Input: part model. Units: mm. Frame: model coordinates. Face numbers are marked on the shaded views. A direction names the side the tool comes from. Coordinates: 2 decimals unless noted, no trailing zeros. Loops run counter-clockwise (first coordinate to the right, second up) from the corner with the lowest first, then second, coordinate; pieces in that order, holes last.
```python
from build123d import *

# Parameters (mm, degrees)
SKETCH1_R            = 3.5
SKETCH1_R_2          = 8
BOSS_EXTRUDE1_DEPTH  = 10
CUT_EXTRUDE1_DEPTH   = 5
FILLET1_R            = 2
SKETCH3_R            = 12.5
CUT_EXTRUDE2_DEPTH   = 10
FILLET1_OF_MIRROR1_R = 2
SKETCH6_R            = 3
CUT_EXTRUDE3_DEPTH   = 10


with BuildPart() as part:
    # Sketch1 → Boss-Extrude1 (new, symmetric)
    # profile 1 of 2: a face of its own
    with BuildSketch(Plane(origin=(0, 0, 0), x_dir=(0, 0, -1), z_dir=(1, 0, 0))):
        with BuildLine():
            ThreePointArc((-46, 62.5), (0, 108.5), (46, 62.5))
            Line((46, 62.5), (46, -62.5))
            Line((46, -62.5), (-46, -62.5))
            Line((-46, -62.5), (-46, 62.5))
        make_face()
        with Locations((-33.774990748, 82)):
            Circle(SKETCH1_R, mode=Mode.SUBTRACT)
        with Locations((-33.774990748, 43)):
            Circle(SKETCH1_R, mode=Mode.SUBTRACT)
        with Locations((0, 23.5)):
            Circle(SKETCH1_R, mode=Mode.SUBTRACT)
        with Locations((33.774990748, 43)):
            Circle(SKETCH1_R, mode=Mode.SUBTRACT)
        with Locations((33.774990748, 82)):
            Circle(SKETCH1_R, mode=Mode.SUBTRACT)
        with Locations((0, 62.5)):
            Circle(SKETCH1_R_2, mode=Mode.SUBTRACT)
        with Locations((0, 101.5)):
            Circle(SKETCH1_R, mode=Mode.SUBTRACT)
        with BuildLine():
            ThreePointArc((-25.103448276, 16.960820334), (-31.051285766, 16.872502771), (-34, 11.706299603))
            Line((-34, 11.706299603), (-34, -44.5))
            ThreePointArc((-34, -44.5), (-32.242640687, -48.742640687), (-28, -50.5))
            Line((-28, -50.5), (28, -50.5))
            ThreePointArc((28, -50.5), (32.242640687, -48.742640687), (34, -44.5))
            Line((34, -44.5), (34, 11.706299603))
            ThreePointArc((34, 11.706299603), (31.051285766, 16.872502771), (25.103448276, 16.960820334))
            ThreePointArc((25.103448276, 16.960820334), (0, 10.5), (-25.103448276, 16.960820334))
        make_face(mode=Mode.SUBTRACT)
    # profile 2 of 2: a face of its own
    with BuildSketch(Plane(origin=(0, 0, 0), x_dir=(0, 0, -1), z_dir=(1, 0, 0))):
        with BuildLine():
            ThreePointArc((-25.103448276, 16.960820334), (0, 10.5), (25.103448276, 16.960820334))
            ThreePointArc((25.103448276, 16.960820334), (31.051285766, 16.872502771), (34, 11.706299603))
            Line((34, 11.706299603), (34, -44.5))
            ThreePointArc((34, -44.5), (32.242640687, -48.742640687), (28, -50.5))
            Line((28, -50.5), (-28, -50.5))
            ThreePointArc((-28, -50.5), (-32.242640687, -48.742640687), (-34, -44.5))
            Line((-34, -44.5), (-34, 11.706299603))
            ThreePointArc((-34, 11.706299603), (-31.051285766, 16.872502771), (-25.103448276, 16.960820334))
        make_face()
    extrude(amount=BOSS_EXTRUDE1_DEPTH, both=True)

    # Sketch2 → Cut-Extrude1 (cut)
    with BuildSketch(Plane(origin=(10, 0, 0), x_dir=(0, 0, -1), z_dir=(1, 0, 0))):
        with BuildLine():
            ThreePointArc((-25.103448276, 16.960820334), (0, 10.5), (25.103448276, 16.960820334))
            ThreePointArc((25.103448276, 16.960820334), (31.051285766, 16.872502771), (34, 11.706299603))
            Line((34, 11.706299603), (34, -44.5))
            ThreePointArc((34, -44.5), (32.242640687, -48.742640687), (28, -50.5))
            Line((28, -50.5), (-28, -50.5))
            ThreePointArc((-28, -50.5), (-32.242640687, -48.742640687), (-34, -44.5))
            Line((-34, -44.5), (-34, 11.706299603))
            ThreePointArc((-34, 11.706299603), (-31.051285766, 16.872502771), (-25.103448276, 16.960820334))
        make_face()
    cut_extrude1 = extrude(amount=-CUT_EXTRUDE1_DEPTH, mode=Mode.SUBTRACT)

    # Fillet1
    fillet1_edges = [part.edges().sort_by_distance(p)[0] for p in [
        (5, -16.396850198, -34),
        (5, 16.872502771, 31.051285766),
        (5, 10.5, 0),
        (5, 16.872502771, -31.051285766),
        (5, -48.742640687, -32.242640687),
        (5, -50.5, 0),
        (5, -48.742640687, 32.242640687),
        (5, -16.396850198, 34),
    ]]
    fillet(fillet1_edges, radius=FILLET1_R)

    # Sketch3 → Cut-Extrude2 (cut)
    with BuildSketch(Plane(origin=(10, 0, 0), x_dir=(0, 0, -1), z_dir=(1, 0, 0))):
        with Locations((0, 62.5)):
            Circle(SKETCH3_R)
    extrude(amount=-CUT_EXTRUDE2_DEPTH, mode=Mode.SUBTRACT)

    # Mirror1: Cut-Extrude1 across plane
    add(cut_extrude1.mirror(Plane(origin=(0, 0, 0), x_dir=(0, 0, 1), z_dir=(1, 0, 0))), mode=Mode.SUBTRACT)

    # Fillet1 of Mirror1
    fillet1_of_mirror1_edges = [part.edges().sort_by_distance(p)[0] for p in [
        (-5, -16.396850198, -34),
        (-5, 16.872502771, 31.051285766),
        (-5, 10.5, 0),
        (-5, 16.872502771, -31.051285766),
        (-5, -48.742640687, -32.242640687),
        (-5, -50.5, 0),
        (-5, -48.742640687, 32.242640687),
        (-5, -16.396850198, 34),
    ]]
    fillet(fillet1_of_mirror1_edges, radius=FILLET1_OF_MIRROR1_R)

    # Sketch6 → Cut-Extrude3 (cut)
    with BuildSketch(Plane.XZ.offset(62.5)):
        with Locations(Location((0, 30, 0), (0, 0, 270))):
            Circle(SKETCH6_R)
        with Locations(Location((0, -30, 0), (0, 0, 270))):
            Circle(SKETCH6_R)
    extrude(amount=-CUT_EXTRUDE3_DEPTH, mode=Mode.SUBTRACT)


solid = part.part
```
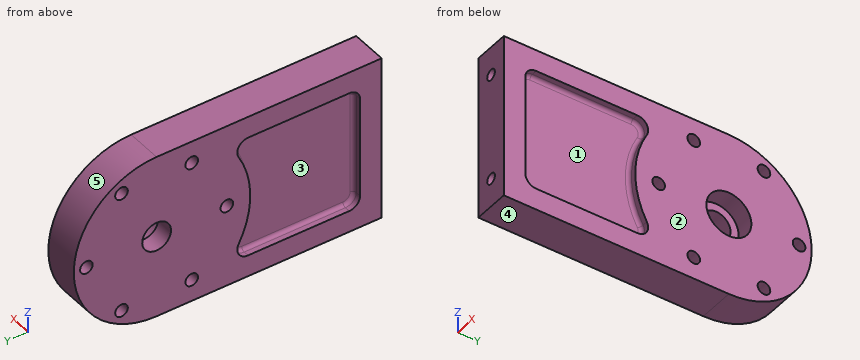
Item 1: Contact query for flat-ended pins moving along their axis: P1, Ø1.5, axis at x = 8, y = 76, coming from the +Z side; P2, Ø20, axis at y = 62.5, z = 0, coming from the +X side; P3, Ø8, axis at y = -30.5, z = -24.5, coming from the +X side. Output: stop coordinate, or through.
Result:
P1: stops at z = 44.2
P2: stops at x = 0
P3: stops at x = 5
Item 2: Mould query, pull axis Y, two halves, no side actions, for the marked faces 3, 4 and 5. Classes: +Y half, -Y half, draft (parallel to the pull), parting line (faces both ways), or undercut.
Result:
face 3: undercut
face 4: draft
face 5: +Y half
Item 3: Line query: L1, parallel to Y at x = 3.75, z = 0; L2, parallel to Y at x = 6, z = -31.5; L3, parallel to Z at x = 8, y = 81. Output: solid intervals per line, ascending.
Result:
L1: y = -62.5 to 20, 27 to 50, 75 to 98, 105 to 108.5
L2: y = -62.5 to -49.04, 16.25 to 40.34, 45.66 to 79.34, 84.66 to 96.02
L3: z = -42.12 to -37.13, -30.42 to 30.42, 37.13 to 42.12
Item 4: Reachability of the marked faces 1 and 2 from +Z, -Z, +X, -X, +Y, -Y: full face, straight path, thin tool, end or side. Return the list, or none.
Result:
face 1: +X
face 2: +Z, -Z, +X, +Y, -Y
Item 5: Section query D-D (y = 101.5). Output: boundary loops of the cut face in (x, z).
Result:
outline: (-10, -24.39) - (10, -24.39) - (10, -3.5) - (-10, -3.5) - close; (-10, 3.5) - (10, 3.5) - (10, 24.39) - (-10, 24.39) - close
Item 6: Section query A-A (z = 0). Count the separate pieces of the cut face and the enclosed holes in it, then the cut area to 3 significant figures.
Result:
separate pieces: 4
enclosed holes: 0
area: 2,120 mm2
Item 7: Section query C-C (y = -13). Output: boundary loops of the cut face in (x, z), then the cut area to 3 significant figures.
Result:
outline: (-10, -46) - (10, -46) - (10, -34) - (7, -34) arc R2 cw to (5, -32) - (5, 32) arc R2 cw to (7, 34) - (10, 34) - (10, 46) - (-10, 46) - (-10, 34) - (-7, 34) arc R2 cw to (-5, 32) - (-5, -32) arc R2 cw to (-7, -34) - (-10, -34) - close
area: 1,160 mm2
Item 8: Section query B-B (y = 43). Output: boundary loops of the cut face in (x, z) (3 decimals).
Result:
outline: (-10, -46) - (10, -46) - (10, -37.275) - (-10, -37.275) - close; (-10, -30.275) - (10, -30.275) - (10, 30.275) - (-10, 30.275) - close; (-10, 37.275) - (10, 37.275) - (10, 46) - (-10, 46) - close
